For this review, take the finished solid that the model builds, in its own axes (mm). Face numbers are marked on the shaded views. A direction names the side the tool comes from. Give positions to 0.01 mm unless a question says otherwise; leave off trailing zeros. Loops run counter-clockwise (first coordinate to the right, second up) from the corner with the lowest first, then second, coordinate; pieces in that order, holes last. Notation, with made-up numbers: (6.25, 37.5) - (18.25, 37.5) arc R18 cw to (18.25, 45.5) - close; hole circle Ø2 at (-13.75, 55). An arc over 180 degrees is marked (long way). Answer in a Markdown table with one row per item.
Autodesk Inventor part; units mm, degrees
ref_plane "YZ Plane" through (0, 0, 0) normal (1, 0, 0) x (0, 1, 0)
ref_plane "XZ Plane" through (0, 0, 0) normal (0, 1, 0) x (-1, 0, 0)
ref_plane "XY Plane" through (0, 0, 0) normal (0, 0, 1) x (1, 0, 0)
sketch "Sketch1" plane through (0, 0, 0) normal (0, 0, 1) x (1, 0, 0)
  line L0 (0, 0) -> (60, 0)
  line L1 (60, 0) -> (60, 140)
  line L2 (60, 140) -> (0, 140)
  line L3 (0, 140) -> (0, 0)
  dimension "d0" = 60
  dimension "d1" = 140
extrude "Extrusion1" add sketch "Sketch1" along normal blind 3
sketch "Sketch4" plane through (0, 0, 3) normal (0, 0, 1) x (1, 0, 0)
  point P0 (0, 0)
sketch "Sketch5" plane through (0, 0, 3) normal (0, 0, 1) x (1, 0, 0)
  circle A0 centre (38.0013, 85.4781) radius 1.5
  circle A1 centre (38.0013, 50.4781) radius 1.5
  line L0 (60, 0) -> (60, 140)
  circle A2 centre (46.5013, 67.9781) radius 4.75
  line L1 (60, 0) -> (60, 140)
  line L2 (60, 67.9781) -> (70, 67.9781) construction
  point P0 (0, 0)
  dimension "d11" = 3
extrude "Extrusion4" cut sketch "Sketch5" against normal blind 145
sketch "Sketch6" plane through (0, 0, 0) normal (-1, 0, 0) x (0, 0, 1)
  line L0 (0, 140) -> (0, 0)
  line L1 (3, 0) -> (3, 140)
  line L2 (0, 0) -> (3, 0)
  line L3 (3, 0) -> (3, 140)
  line L4 (3, 140) -> (0, 140)
  line L5 (0, 140) -> (0, 0)
extrude "Extrusion5" add sketch "Sketch6" along normal blind 5
sketch "Sketch7" plane through (60, 140, 3) normal (0, 1, 0) x (1, 0, 0)
  line L0 (-65, 0) -> (-65, 3)
  line L1 (-65, 3) -> (0, 3)
  line L2 (0, 3) -> (0, -17)
  line L3 (0, -17) -> (-65, -17)
  line L4 (-65, -17) -> (-65, 3)
  arc A0 (-28.1699, -4.5) -> (-28.1699, -9.5) centre (-32.5, -7) ccw
  line L5 (-25, -9.5) -> (-25, -4.5)
  line L6 (-40, -4.5) -> (-25, -9.5) construction
  line L7 (-40, -9.5) -> (-25, -4.5) construction
  line L8 (-28.1699, -9.5) -> (-25, -9.5)
  line L9 (-25, -4.5) -> (-28.1699, -4.5)
  point P0 (-60, 3)
  dimension "d18" = 65
  dimension "d19" = 20
sketch "Sketch8" plane through (0, 0, 3) normal (0, 0, 1) x (1, 0, 0)
  line L0 (35, 0) -> (35, 140)
  line L1 (35, 140) -> (20, 140)
  line L2 (20, 140) -> (20, 0)
  line L3 (20, 0) -> (35, 0)
  line L4 (35, 0) -> (20, 140) construction
  line L5 (35, 140) -> (20, 0) construction
  line L6 (60, 0) -> (60, 140)
  line L7 (35, 0) -> (175, 0) construction
  point P0 (0, 0)
  point P1 (27.5, 70)
  dimension "d21" = 140
  dimension "d22" = 90
  dimension "d23" = 15
extrude "Extrusion6" add sketch "Sketch8" along normal blind 14
extrude "Extrusion7" cut sketch "Sketch7" against normal blind 140 contours L9 L5 L8 A0
sketch "Sketch9" plane through (0, 0, 3) normal (0, 0, 1) x (1, 0, 0)
  point P0 (0, 0)
properties part number "Rack Base"
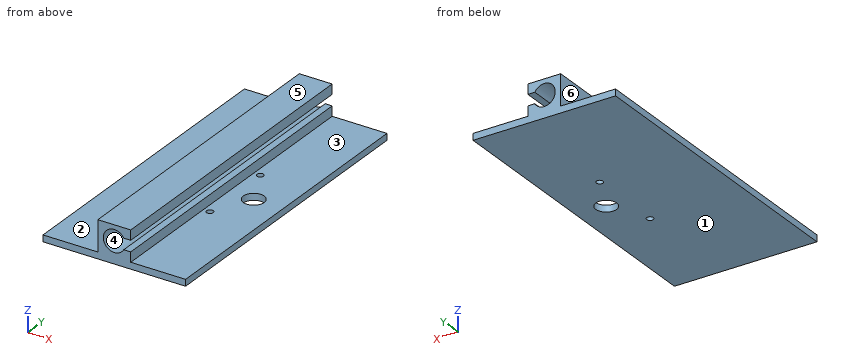
1. For the marked faces 1, 2 and 3, list the 3-axis set-ups (+Z, -Z, +X, -X, +Y, -Y) from which the entire face can be reached by the end or side of a thin tool; tool diameter is ignored.
Values:
| item | result |
|---|---|
| face 1 | -Z, +X, -X, +Y, -Y |
| face 2 | +Z, -X, +Y, -Y |
| face 3 | +Z, +X, +Y, -Y |
2. We need section A-A, the plane x = 27.5. Give the boundary of the cut face in (y, z), and give its area (3 significant figures).
Values:
| item | result |
|---|---|
| outline | (0, 0) - (140, 0) - (140, 5) - (0, 5) - close; (0, 15) - (140, 15) - (140, 17) - (0, 17) - close |
| area | 980 mm^2 |
3. We need section C-C, the plane z = 10. Give the boundary of the cut face in (x, y), and give its area (3 significant figures).
Values:
| item | result |
|---|---|
| outline | (20, 0) - (22.5, 0) - (22.5, 140) - (20, 140) - close |
| area | 350 mm^2 |
4. Clearance check with flat-ended pins moving along their axes: pin 1 (1.6 mm diameter, centred on x = 34, y = 104, fed in from -Z); pin 2 (1.5 mm diameter, centred on x = 37.5, z = 4.5, fed in from -Y); pin 3 (2 mm diameter, centred on y = 47, z = 10.5, fed in from +X); pin 4 (12.5 mm diameter, centred on x = 46.5, y = 67.98, fed in from +Z). State where each tip first meets the part, or that it passes through.
Values:
| item | result |
|---|---|
| pin 1 | stops at z = 0 |
| pin 2 | passes through |
| pin 3 | stops at x = 22.73 |
| pin 4 | stops at z = 3 |
5. Mouldability with a two-part tool opening along X and no side actions: class the marked faces 4, 5 and 6 as released by +X, released by -X, zero draft, split by the parting line, or undercut.
Values:
| item | result |
|---|---|
| face 4 | undercut |
| face 5 | zero draft |
| face 6 | released by -X |
6. We need section D-D, the plane x = 56.5. Give the boundary of the cut face in (y, z).
Values:
| item | result |
|---|---|
| outline | (0, 0) - (140, 0) - (140, 3) - (0, 3) - close |
7. Wall thickness on line 1 (Z direction, x = 27, y = 31); line 2 (Z direction, x = 32, y = 31); line 3 (Z direction, x = 14, y = 43): over which ranges is each line inside the solid? List them lowest first. Write a range as [from, to].
Values:
| item | result |
|---|---|
| line 1 | z = [0, 5.03], [14.97, 17] |
| line 2 | z = [0, 7.5], [12.5, 17] |
| line 3 | z = [0, 3] |
8. We need section B-B, the plane y = 12. Give the boundary of the cut face in (x, z), and give its area (3 significant figures).
Values:
| item | result |
|---|---|
| outline | (-5, 0) - (60, 0) - (60, 3) - (35, 3) - (35, 7.5) - (31.83, 7.5) arc R5 cw (long way) to (31.83, 12.5) - (35, 12.5) - (35, 17) - (20, 17) - (20, 3) - (-5, 3) - close |
| area | 313 mm^2 |
